The model under review builds one solid part; all positions refer to its coordinate system, in mm. Round coordinates to 2 decimals unless told otherwise and drop trailing zeros. Write each loop counter-clockwise with the first axis right and the second up, starting at its lowest first coordinate (ties: lowest second). Pieces come first, ordered by that corner, then holes. Notation, with made-up numbers: (76, 22.25) -> (94, 22.25) arc R31 ccw to (94, 49.25) -> close; hole circle Ø10 at (34, 61.25). An arc over 180 degrees is marked (long way). Use CSV: the item, a comma, the result in double quotes. Start each with the question number.
1) Take a section at B-B, the plane y = -27. State how many separate pieces and enclosed holes the cut face has, then the cut area to 3 significant figures.
2) Wall thickness on probe 1 along X at (y, z) = (-14, -58); probe 2 along X at (y, z) = (-23.5, 15.5) (3 decimals); probe 3 along Z at (x, y) = (36, -10): over which ranges is each line inside the solid? List them lowest first. Write a range as [from, to].
3) Take a section at A-A, the plane z = 0. Give the boundary of the cut face in (x, y) (3 decimals), then the cut area to 3 significant figures.
4) For pin 1 Ø14 at (x, y) = (-52.5, -26.5) entering from -Z; pin 2 Ø10 at (x, y) = (45.5, -25) entering from -Z; pin 3 Ø3 at (x, z) = (45.5, 83.5) entering from +Y; pin 4 Ø1.9 at (x, y) = (-60, -14.5) entering from +Z, all flat-tipped, find the tip position at first contact; note any pin that passes through.
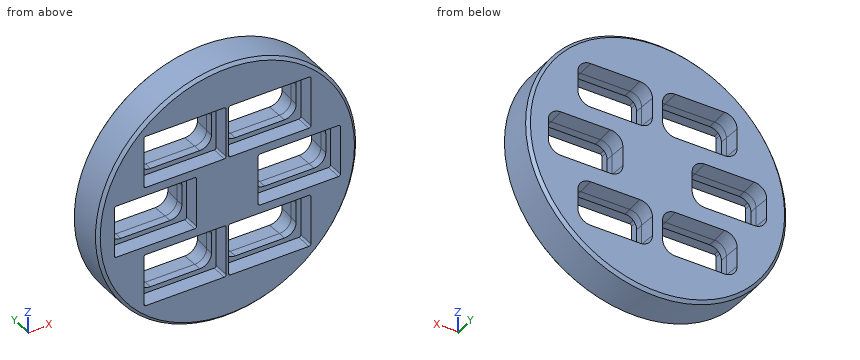
from build123d import *

# Parameters (mm, degrees)
F0_R     = 104.775
F1_DEPTH = 31.75
F2_SIZE  = 2.3622
F3_SIZE  = 2.3622
F5_DEPTH = 12.7
F7_DEPTH = 19.051
F8_SIZE2 = 12.7
F8_SIZE  = 0.6655787969


with BuildPart() as f1:
    # F0 (on Front) → F1 (new body)
    with BuildSketch(Plane.XZ):
        Circle(F0_R)
    extrude(amount=F1_DEPTH)

    # F2
    f2_edges = [f1.edges().sort_by_distance(p)[0] for p in [
        (-104.775, -31.75, 0),
    ]]
    chamfer(f2_edges, length=F2_SIZE)

    # F3
    f3_edges = [f1.edges().sort_by_distance(p)[0] for p in [
        (-104.775, 0, 0),
    ]]
    chamfer(f3_edges, length=F3_SIZE)

    # F4 (on face) → F5 (cut)
    with BuildSketch(Plane.XZ.offset(31.75)):
        with BuildLine():
            ThreePointArc((-24.765, 19.6977), (-25.226248241, 20.811251759), (-26.3398, 21.2725))
            Line((-26.3398, 21.2725), (-89.535, 21.2725))
            ThreePointArc((-89.535, 21.2725), (-90.648551759, 20.811251759), (-91.1098, 19.6977))
            Line((-91.1098, 19.6977), (-91.1098, -19.6977))
            ThreePointArc((-91.1098, -19.6977), (-90.648551759, -20.811251759), (-89.535, -21.2725))
            Line((-89.535, -21.2725), (-26.3398, -21.2725))
            ThreePointArc((-26.3398, -21.2725), (-25.226248241, -20.811251759), (-24.765, -19.6977))
            Line((-24.765, -19.6977), (-24.765, 19.6977))
        make_face()
        with BuildLine():
            ThreePointArc((91.1098, 19.6977), (90.648551759, 20.811251759), (89.535, 21.2725))
            Line((89.535, 21.2725), (26.3398, 21.2725))
            ThreePointArc((26.3398, 21.2725), (25.226248241, 20.811251759), (24.765, 19.6977))
            Line((24.765, 19.6977), (24.765, -19.6977))
            ThreePointArc((24.765, -19.6977), (25.226248241, -20.811251759), (26.3398, -21.2725))
            Line((26.3398, -21.2725), (89.535, -21.2725))
            ThreePointArc((89.535, -21.2725), (90.648551759, -20.811251759), (91.1098, -19.6977))
            Line((91.1098, -19.6977), (91.1098, 19.6977))
        make_face()
        with BuildLine():
            ThreePointArc((-0.9525, 68.9102), (-1.413748241, 70.023751759), (-2.5273, 70.485))
            Line((-2.5273, 70.485), (-65.7225, 70.485))
            ThreePointArc((-65.7225, 70.485), (-66.836051759, 70.023751759), (-67.2973, 68.9102))
            Line((-67.2973, 68.9102), (-67.2973, 29.5148))
            ThreePointArc((-67.2973, 29.5148), (-66.836051759, 28.401248241), (-65.7225, 27.94))
            Line((-65.7225, 27.94), (-2.5273, 27.94))
            ThreePointArc((-2.5273, 27.94), (-1.413748241, 28.401248241), (-0.9525, 29.5148))
            Line((-0.9525, 29.5148), (-0.9525, 68.9102))
        make_face()
        with BuildLine():
            Line((65.7098, 70.485), (2.5146, 70.485))
            ThreePointArc((2.5146, 70.485), (1.401048241, 70.023751759), (0.9398, 68.9102))
            Line((0.9398, 68.9102), (0.9398, 29.5148))
            ThreePointArc((0.9398, 29.5148), (1.401048241, 28.401248241), (2.5146, 27.94))
            Line((2.5146, 27.94), (65.7098, 27.94))
            ThreePointArc((65.7098, 27.94), (66.823351759, 28.401248241), (67.2846, 29.5148))
            Line((67.2846, 29.5148), (67.2846, 68.9102))
            ThreePointArc((67.2846, 68.9102), (66.823351759, 70.023751759), (65.7098, 70.485))
        make_face()
        with BuildLine():
            ThreePointArc((-0.9525, -29.5148), (-1.413748241, -28.401248241), (-2.5273, -27.94))
            Line((-2.5273, -27.94), (-65.7225, -27.94))
            ThreePointArc((-65.7225, -27.94), (-66.836051759, -28.401248241), (-67.2973, -29.5148))
            Line((-67.2973, -29.5148), (-67.2973, -68.9102))
            ThreePointArc((-67.2973, -68.9102), (-66.836051759, -70.023751759), (-65.7225, -70.485))
            Line((-65.7225, -70.485), (-2.5273, -70.485))
            ThreePointArc((-2.5273, -70.485), (-1.413748241, -70.023751759), (-0.9525, -68.9102))
            Line((-0.9525, -68.9102), (-0.9525, -29.5148))
        make_face()
        with BuildLine():
            Line((65.7098, -27.94), (2.5146, -27.94))
            ThreePointArc((2.5146, -27.94), (1.401048241, -28.401248241), (0.9398, -29.5148))
            Line((0.9398, -29.5148), (0.9398, -68.9102))
            ThreePointArc((0.9398, -68.9102), (1.401048241, -70.023751759), (2.5146, -70.485))
            Line((2.5146, -70.485), (65.7098, -70.485))
            ThreePointArc((65.7098, -70.485), (66.823351759, -70.023751759), (67.2846, -68.9102))
            Line((67.2846, -68.9102), (67.2846, -29.5148))
            ThreePointArc((67.2846, -29.5148), (66.823351759, -28.401248241), (65.7098, -27.94))
        make_face()
    extrude(amount=-F5_DEPTH, mode=Mode.SUBTRACT)

    # F6 (on face) → F7 (cut, through all)
    with BuildSketch(Plane.XZ.offset(19.05)):
        with BuildLine():
            ThreePointArc((-4.7625, 57.15), (-7.5523079092, 63.8851920908), (-14.2875, 66.675))
            Line((-14.2875, 66.675), (-53.9623, 66.675))
            ThreePointArc((-53.9623, 66.675), (-60.6974920908, 63.8851920908), (-63.4873, 57.15))
            Line((-63.4873, 57.15), (-63.4873, 41.275))
            ThreePointArc((-63.4873, 41.275), (-60.6974920908, 34.5398079092), (-53.9623, 31.75))
            Line((-53.9623, 31.75), (-14.2875, 31.75))
            ThreePointArc((-14.2875, 31.75), (-7.5523079092, 34.5398079092), (-4.7625, 41.275))
            Line((-4.7625, 41.275), (-4.7625, 57.15))
        make_face()
        with BuildLine():
            ThreePointArc((53.9623, 31.75), (60.6974920908, 34.5398079092), (63.4873, 41.275))
            Line((63.4873, 41.275), (63.4873, 57.15))
            ThreePointArc((63.4873, 57.15), (60.6974920908, 63.8851920908), (53.9623, 66.675))
            Line((53.9623, 66.675), (14.2875, 66.675))
            ThreePointArc((14.2875, 66.675), (7.5523079092, 63.8851920908), (4.7625, 57.15))
            Line((4.7625, 57.15), (4.7625, 41.275))
            ThreePointArc((4.7625, 41.275), (7.5523079092, 34.5398079092), (14.2875, 31.75))
            Line((14.2875, 31.75), (53.9623, 31.75))
        make_face()
        with BuildLine():
            ThreePointArc((4.7625, -57.15), (7.5523079092, -63.8851920908), (14.2875, -66.675))
            Line((14.2875, -66.675), (53.9623, -66.675))
            ThreePointArc((53.9623, -66.675), (60.6974920908, -63.8851920908), (63.4873, -57.15))
            Line((63.4873, -57.15), (63.4873, -41.275))
            ThreePointArc((63.4873, -41.275), (60.6974920908, -34.5398079092), (53.9623, -31.75))
            Line((53.9623, -31.75), (14.2875, -31.75))
            ThreePointArc((14.2875, -31.75), (7.5523079092, -34.5398079092), (4.7625, -41.275))
            Line((4.7625, -41.275), (4.7625, -57.15))
        make_face()
        with BuildLine():
            ThreePointArc((-63.4873, -57.15), (-60.6974920908, -63.8851920908), (-53.9623, -66.675))
            Line((-53.9623, -66.675), (-14.2875, -66.675))
            ThreePointArc((-14.2875, -66.675), (-7.5523079092, -63.8851920908), (-4.7625, -57.15))
            Line((-4.7625, -57.15), (-4.7625, -41.275))
            ThreePointArc((-4.7625, -41.275), (-7.5523079092, -34.5398079092), (-14.2875, -31.75))
            Line((-14.2875, -31.75), (-53.9623, -31.75))
            ThreePointArc((-53.9623, -31.75), (-60.6974920908, -34.5398079092), (-63.4873, -41.275))
            Line((-63.4873, -41.275), (-63.4873, -57.15))
        make_face()
        with BuildLine():
            ThreePointArc((-28.575, 7.9375), (-31.3648079092, 14.6726920908), (-38.1, 17.4625))
            Line((-38.1, 17.4625), (-77.7748, 17.4625))
            ThreePointArc((-77.7748, 17.4625), (-84.5099920908, 14.6726920908), (-87.2998, 7.9375))
            Line((-87.2998, 7.9375), (-87.2998, -7.9375))
            ThreePointArc((-87.2998, -7.9375), (-84.5099920908, -14.6726920908), (-77.7748, -17.4625))
            Line((-77.7748, -17.4625), (-38.1, -17.4625))
            ThreePointArc((-38.1, -17.4625), (-31.3648079092, -14.6726920908), (-28.575, -7.9375))
            Line((-28.575, -7.9375), (-28.575, 7.9375))
        make_face()
        with BuildLine():
            Line((77.7748, 17.4625), (38.1, 17.4625))
            ThreePointArc((38.1, 17.4625), (31.3648079092, 14.6726920908), (28.575, 7.9375))
            Line((28.575, 7.9375), (28.575, -7.9375))
            ThreePointArc((28.575, -7.9375), (31.3648079092, -14.6726920908), (38.1, -17.4625))
            Line((38.1, -17.4625), (77.7748, -17.4625))
            ThreePointArc((77.7748, -17.4625), (84.5099920908, -14.6726920908), (87.2998, -7.9375))
            Line((87.2998, -7.9375), (87.2998, 7.9375))
            ThreePointArc((87.2998, 7.9375), (84.5099920908, 14.6726920908), (77.7748, 17.4625))
        make_face()
    extrude(amount=-F7_DEPTH, mode=Mode.SUBTRACT)

    # F8
    f8_edges = [f1.edges().sort_by_distance(p)[0] for p in [
        (34.1249, 0, 66.675),
        (-34.1249, 0, 66.675),
        (-57.9374, 0, 17.4625),
        (57.9374, 0, 17.4625),
        (34.1249, 0, -31.75),
        (-34.1249, 0, -31.75),
    ]]
    f8_side = f1.faces().sort_by_distance((0, 0, 0))[0]
    chamfer(f8_edges, length=F8_SIZE, length2=F8_SIZE2, reference=f8_side)


solid = f1.part
Values found:
1,separate pieces,"1"
1,enclosed holes,"6"
1,area,"17,600 mm²"
2,probe 1,"[-87.26, -63.45], [-4.8, 4.8], [63.45, 87.26]"
2,probe 2,"[-103.622, -91.11], [-24.765, 24.765], [91.11, 103.622]"
2,probe 3,"[-98.4, -66.82], [-31.61, -17.37], [17.37, 31.61], [66.82, 98.4]"
3,outline,"(-104.775, -29.388) -> (-102.413, -31.75) -> (-91.11, -31.75) -> (-91.11, -19.05) -> (-87.3, -19.05) -> (-87.3, -12.7) -> (-87.965, 0) -> (-102.413, 0) -> (-104.775, -2.362) -> close; (-28.575, -19.05) -> (-24.765, -19.05) -> (-24.765, -31.75) -> (24.765, -31.75) -> (24.765, -19.05) -> (28.575, -19.05) -> (28.575, -12.7) -> (27.909, 0) -> (-27.909, 0) -> (-28.575, -12.7) -> close; (87.3, -19.05) -> (91.11, -19.05) -> (91.11, -31.75) -> (102.413, -31.75) -> (104.775, -29.388) -> (104.775, -2.362) -> (102.413, 0) -> (87.965, 0) -> (87.3, -12.7) -> close"
3,area,"2,700 mm²"
4,pin 1,"z = -94.38"
4,pin 2,"z = -96.63"
4,pin 3,"y = 0"
4,pin 4,"z = 86.55"
